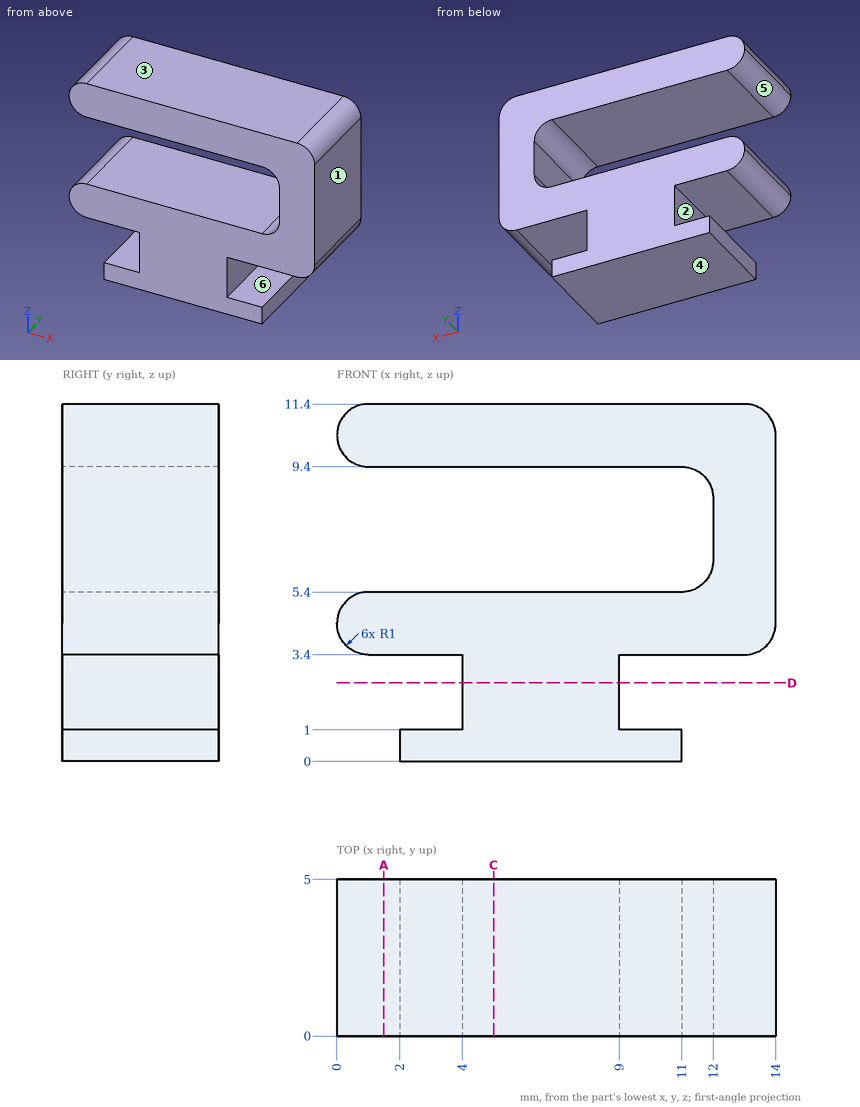
Job drawing, mm, ordinate dimensions from the low corner. One solid piece. A direction names the side the tool comes from. Round coordinates to 2 decimals unless told otherwise and drop trailing zeros. Loops run counter-clockwise (first coordinate to the right, second up) from the corner with the lowest first, then second, coordinate; pieces in that order, holes last. Notation, with made-up numbers: (14, 72) -> (69, 72) arc R24 cw to (69, 95) -> close; hole circle Ø5 at (3, -35). An arc over 180 degrees is marked (long way). Use a Markdown table: item, result.
1) Cut at A-A, the plane x = 1.5. List the corners of the cut face in (y, z).
The answers:
| item | result |
|---|---|
| outline | (0, 3.4) -> (5, 3.4) -> (5, 5.4) -> (0, 5.4) -> close; (0, 9.4) -> (5, 9.4) -> (5, 11.4) -> (0, 11.4) -> close |
2) Drop flat-ended pins along their axis: pin 1 Ø1.5 at (y, z) = (1, 2.5) entering from -X; pin 2 Ø1.2 at (y, z) = (1.5, 2.5) entering from +X; pin 3 Ø1.6 at (y, z) = (1.5, 7) entering from -X. Give the stop position or say it passes through.
The answers:
| item | result |
|---|---|
| pin 1 | stops at x = 4 |
| pin 2 | stops at x = 9 |
| pin 3 | stops at x = 11.98 |
3) Tool access for the marked faces 4, 5 and 6: list every direction of +Z, -Z, +X, -X, +Y, -Y with a clear straight run to the whole face (end or side of a thin tool).
The answers:
| item | result |
|---|---|
| face 4 | -Z, +X, -X, +Y, -Y |
| face 5 | -X, +Y, -Y |
| face 6 | +X, +Y, -Y |
4) Cut at C-C, the plane x = 5. List the corners of the cut face in (y, z), and give its area (3 significant figures).
The answers:
| item | result |
|---|---|
| outline | (0, 0) -> (5, 0) -> (5, 5.4) -> (0, 5.4) -> close; (0, 9.4) -> (5, 9.4) -> (5, 11.4) -> (0, 11.4) -> close |
| area | 37.0 mm2 |
5) Cut at D-D, the plane z = 2.5. List the corners of the cut face in (x, y).
The answers:
| item | result |
|---|---|
| outline | (4, 0) -> (9, 0) -> (9, 5) -> (4, 5) -> close |
6) Probe line 1 (Z direction, x = 10.75, y = 3.65); line 2 (Z direction, x = 1.75, y = 1.85); line 3 (Z direction, x = 6.75, y = 1). List the from-to ranges inside material, lowest first. Write a range as [from, to].
The answers:
| item | result |
|---|---|
| line 1 | z = [0, 1], [3.4, 5.4], [9.4, 11.4] |
| line 2 | z = [3.4, 5.4], [9.4, 11.4] |
| line 3 | z = [0, 5.4], [9.4, 11.4] |
7) Pull direction Z, two halves, no side cores. Call the marked faces 1, 2 and 3: pulls with the +Z half, pulls with the -Z half, needs draft (parallel to the pull), parting line crosses it, or undercut.
The answers:
| item | result |
|---|---|
| face 1 | needs draft |
| face 2 | undercut |
| face 3 | pulls with the +Z half |
